Verification items for the finished model (mm, model axes). A direction names the side the tool comes from. Give positions to 0.01 mm unless a question says otherwise; leave off trailing zeros. Write each loop counter-clockwise with the first axis right and the second up, starting at its lowest first coordinate (ties: lowest second). Pieces come first, ordered by that corner, then holes.
from build123d import *

# Parameters (mm, degrees)
SKETCH2_R           = 20.701
BOSS_EXTRUDE1_DEPTH = 19.05
CUT_EXTRUDE2_DEPTH  = 12.7
SKETCH15_R          = 22.225
BOSS_EXTRUDE2_DEPTH = 3.175


with BuildPart() as part:
    # Sketch2 → Boss-Extrude1 (new body)
    with BuildSketch(Plane(origin=(0, 0, 0), x_dir=(1, 0, 0), z_dir=(0, 1, 0))):
        with Locations(Location((0, 0, 0), (0, 0, 90))):
            Circle(SKETCH2_R)
        with BuildLine():
            Line((-13.081, 3.175), (-8.059107313, -1.349826056))
            ThreePointArc((-8.059107313, -1.349826056), (0, -4.445), (8.059107313, -1.349826056))
            Line((8.059107313, -1.349826056), (13.081, 3.175))
            ThreePointArc((13.081, 3.175), (13.146371637, 4.430535164), (11.890836473, 4.495906802))
            Line((11.890836473, 4.495906802), (6.868943786, -0.028919255))
            ThreePointArc((6.868943786, -0.028919255), (0, -2.667), (-6.868943786, -0.028919255))
            Line((-6.868943786, -0.028919255), (-11.890836473, 4.495906802))
            ThreePointArc((-11.890836473, 4.495906802), (-13.146371637, 4.430535164), (-13.081, 3.175))
        make_face(mode=Mode.SUBTRACT)
    extrude(amount=BOSS_EXTRUDE1_DEPTH)

    # Sketch14 → Cut-Extrude2 (cut)
    with BuildSketch(Plane(origin=(0, 19.05, 0), x_dir=(1, 0, 0), z_dir=(0, 1, 0))):
        with BuildLine():
            Line((8.603182068, -1.953669166), (13.625074755, 2.571156891))
            ThreePointArc((13.625074755, 2.571156891), (13.750214746, 4.97460992), (11.346761717, 5.099749911))
            Line((11.346761717, 5.099749911), (6.32486903, 0.574923855))
            ThreePointArc((6.32486903, 0.574923855), (0, -1.8542), (-6.32486903, 0.574923855))
            Line((-6.32486903, 0.574923855), (-11.346761717, 5.099749911))
            ThreePointArc((-11.346761717, 5.099749911), (-13.750214746, 4.97460992), (-13.625074755, 2.571156891))
            Line((-13.625074755, 2.571156891), (-8.603182068, -1.953669166))
            ThreePointArc((-8.603182068, -1.953669166), (0, -5.2578), (8.603182068, -1.953669166))
        make_face()
    extrude(amount=-CUT_EXTRUDE2_DEPTH, mode=Mode.SUBTRACT)

    # Sketch15 → Boss-Extrude2 (add)
    with BuildSketch(Plane.XZ):
        with Locations(Location((0, 0, 0), (0, 0, 270))):
            Circle(SKETCH15_R)
        with BuildLine():
            Line((-13.081, -3.175), (-8.059107313, 1.349826056))
            ThreePointArc((-8.059107313, 1.349826056), (0, 4.445), (8.059107313, 1.349826056))
            Line((8.059107313, 1.349826056), (13.081, -3.175))
            ThreePointArc((13.081, -3.175), (13.146371637, -4.430535164), (11.890836473, -4.495906802))
            Line((11.890836473, -4.495906802), (6.868943786, 0.028919255))
            ThreePointArc((6.868943786, 0.028919255), (0, 2.667), (-6.868943786, 0.028919255))
            Line((-6.868943786, 0.028919255), (-11.890836473, -4.495906802))
            ThreePointArc((-11.890836473, -4.495906802), (-13.146371637, -4.430535164), (-13.081, -3.175))
        make_face(mode=Mode.SUBTRACT)
    extrude(amount=-BOSS_EXTRUDE2_DEPTH)


solid = part.part
Item 1: Sectioned sample at A-A on y = 8.5. Record the cut outline in (x, z), then the cut area to 3 significant figures.
Answer key:
outline: circle Ø41.4 at (0, 0); hole (-13.63, -2.57) arc R1.7 ccw to (-11.35, -5.1) - (-6.32, -0.57) arc R9.45 cw to (6.32, -0.57) - (11.35, -5.1) arc R1.7 ccw to (13.63, -2.57) - (8.6, 1.95) arc R12.85 ccw to (-8.6, 1.95) - close
area: 1,240 mm2
Item 2: Sectioned sample at D-D on z = -16. Record the cut outline in (x, y) (3 decimals).
Answer key:
outline: (-15.426, 0) - (15.426, 0) - (15.426, 3.175) - (13.135, 3.175) - (13.135, 19.05) - (-13.135, 19.05) - (-13.135, 3.175) - (-15.426, 3.175) - close
Item 3: Release check for a two-part mould opening along X. For faces 4 (the face through (0.097, 12.789, 1.854)), 5 (the face through (20.21, 11, 4.49)), 6 (the face through (7, 3.175, -20)) record: released by +X, released by -X, zero draft, split by the parting line, or undercut.
Answer key:
face 4: undercut
face 5: split by the parting line
face 6: zero draft
Item 4: Sectioned sample at B-B on x = 0. Record the cut outline in (y, z) (3 decimals).
Answer key:
outline: (0, -22.225) - (3.175, -22.225) - (3.175, -20.701) - (19.05, -20.701) - (19.05, 1.854) - (6.35, 1.854) - (6.35, 2.667) - (0, 2.667) - close; (0, 4.445) - (6.35, 4.445) - (6.35, 5.258) - (19.05, 5.258) - (19.05, 20.701) - (3.175, 20.701) - (3.175, 22.225) - (0, 22.225) - close
Item 5: Set-up check for faces 1 (the face through (-9.34, 3.13, -2.2)), 2 (the face through (-13.725, 12.789, -5.002)), 3 (the face through (0, 0, 0)): record each of +Z, -Z, +X, -X, +Y, -Y from which the full face is reachable in a straight line by a thin tool's end or side.
Answer key:
face 1: +Y, -Y
face 2: +Y
face 3: +Z, -Z, +X, -X, -Y
Item 6: Scan lines: line 1 along X through (y, z) = (7, -3); line 2 along Z through (x, y) = (-13, 17.5); line 3 along Z through (x, y) = (-1, 4). Record each from-to range of solid material in increasing order.
Answer key:
line 1: x = -20.48 to -13.97, -9.02 to 9.02, 13.97 to 20.48
line 2: z = -16.11 to -5.46, -2.01 to 16.11
line 3: z = -20.68 to 2.62, 4.4 to 20.68
Item 7: Depth check by flat-ended pin: pin 1 (3 mm diameter, centred on x = 4.5, y = 11.5, fed in from +Z); pin 2 (8 mm diameter, centred on x = -11.5, y = 14.5, fed in from +Z); pin 3 (1.5 mm diameter, centred on x = -14, y = 8.5, fed in from +Z) (3 decimals). Enter the tip coordinate at first touch or a pass-through.
Answer key:
pin 1: stops at z = 20.48
pin 2: stops at z = 19.29
pin 3: stops at z = 15.905
